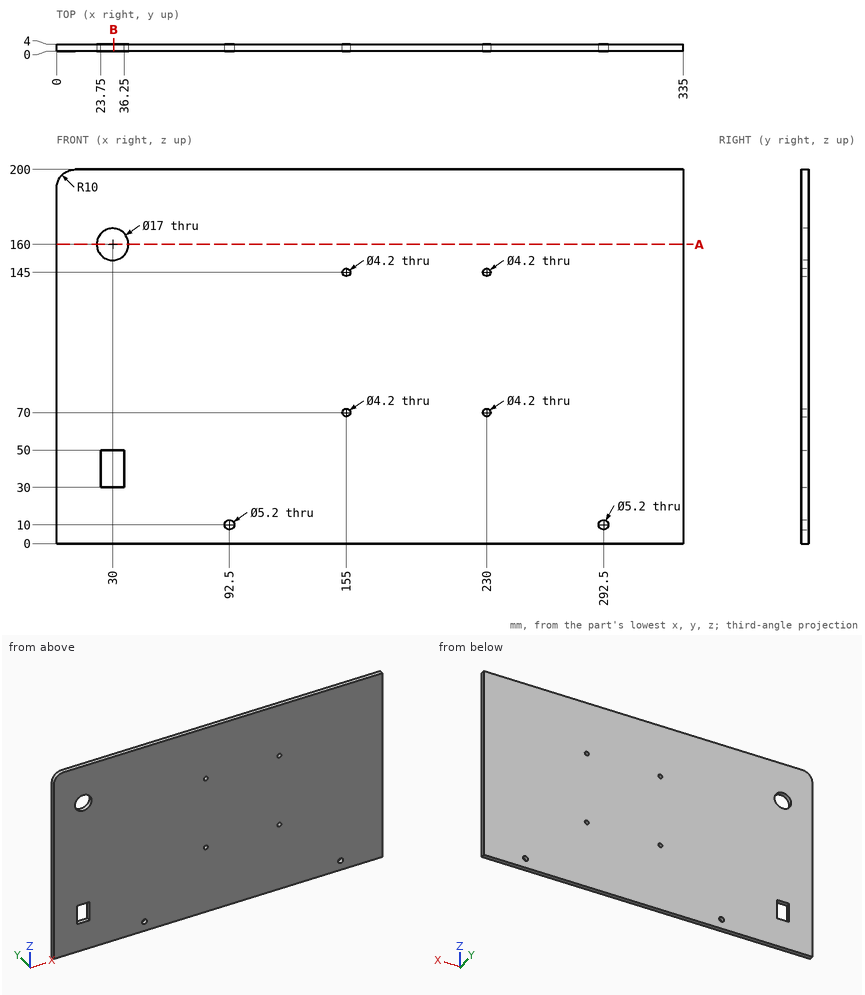
Design review of the part shown in the three views and the two pictorial views. Dimensions are in mm from the part's minimum x, y and z. Round coordinates to 2 decimals unless told otherwise and drop trailing zeros. Loops run counter-clockwise (first coordinate to the right, second up) from the corner with the lowest first, then second, coordinate; pieces in that order, holes last. Notation, with made-up numbers: M 52.5,62.5 L 80.5,62.5 A15 ccw 80.5,80.5 Z; hole C 19,8 d4. An arc over 180 degrees is marked long. Answer as a JSON object with one key per item and string values.
Item 1: Clearance check with a flat-ended pin moving along its axis: P1, Ø3.5, axis at x = 230, z = 145, coming from the +Y side. State where the tip first meets the part, or that it passes through.
Check sheet entries:
{"P1": "through"}
Item 2: For line 1 along X through (y, z) = (2.05, 70); line 2 along Z through (x, y) = (230, 1); line 3 along Z through (x, y) = (30, 0.9), list the stretches that pass through material, from the lowest coordinate up.
Check sheet entries:
{"line 1": "0 to 152.9, 157.1 to 227.9, 232.1 to 335", "line 2": "0 to 67.9, 72.1 to 142.9, 147.1 to 200", "line 3": "0 to 30, 50 to 151.5, 168.5 to 200"}
Item 3: We need section B-B, the plane x = 30.5. State the section outline as (y, z) points, and give its area (3 significant figures).
Check sheet entries:
{"outline": "M 0,0 L 4,0 L 4,30 L 0,30 Z; M 0,50 L 4,50 L 4,151.51 L 0,151.51 Z; M 0,168.49 L 4,168.49 L 4,200 L 0,200 Z", "area": "652 mm2"}
Item 4: We need section A-A, the plane z = 160. State the section outline as (x, y) points.
Check sheet entries:
{"outline": "M 0,0 L 21.5,0 L 21.5,4 L 0,4 Z; M 38.5,0 L 335,0 L 335,4 L 38.5,4 Z"}
